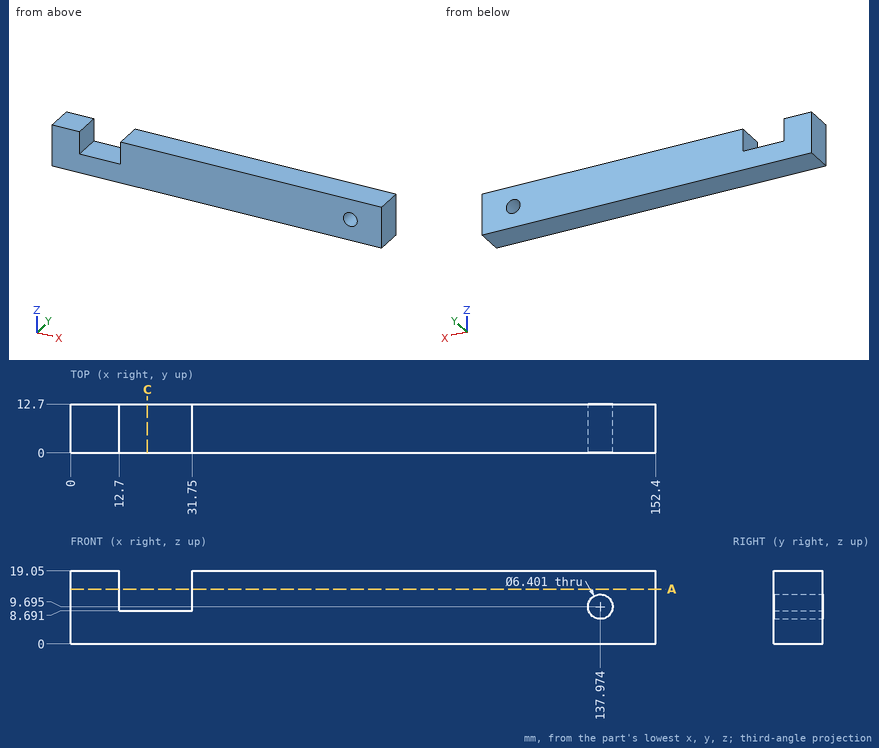
Geometry check sheet. Reference: drawing and pictorial views, mm from the part's lowest x, y, z. Coordinates: 2 decimals unless noted, no trailing zeros. Write each loop counter-clockwise with the first axis right and the second up, starting at its lowest first coordinate (ties: lowest second). Pieces come first, ordered by that corner, then holes. Notation, with made-up numbers: M -16,-26 L 25,-26 A17 cw 25,-6 Z; hole C 27,28 d10. An arc over 180 degrees is marked long. Write item = value, one per line. Start each with the question number.
1. Sectioned sample at A-A (z = 14.25). Record the cut outline in (x, y).
2. Sectioned sample at C-C (x = 20). Record the cut outline in (y, z).
3. Thickness scan on probe 1 along X at (y, z) = (11, 10); probe 2 along X at (y, z) = (7.25, 18.25); probe 3 along Z at (x, y) = (30.5, 4). Record the ranges inside material, lowest first.
The answers:
q1.outline = M 0,0 L 12.7,0 L 12.7,12.7 L 0,12.7 Z; M 31.75,0 L 152.4,0 L 152.4,12.7 L 31.75,12.7 Z
q2.outline = M 0,0 L 12.7,0 L 12.7,8.69 L 0,8.69 Z
q3.probe_1 = 0 to 12.7, 31.75 to 134.79, 141.16 to 152.4
q3.probe_2 = 0 to 12.7, 31.75 to 152.4
q3.probe_3 = 0 to 8.69
